Part model, mm, in its own coordinate system. A direction names the side the tool comes from. Round coordinates to 2 decimals unless told otherwise and drop trailing zeros. Loops run counter-clockwise (first coordinate to the right, second up) from the corner with the lowest first, then second, coordinate; pieces in that order, holes last. Notation, with made-up numbers: M 64.25,-15 L 120.25,-15 A24 ccw 120.25,13 Z; hole C -8,25.5 d4. An arc over 180 degrees is marked long. Put each result on its own line as item: value. Start each with the question number.
1) Slice it at B-B on x = 64.5. Give the cut face in (y, z).
2) Pull direction X, two halves, no side cores. Call faces 1 (the cylindrical face through (-11.797, -7.259, 11.668)), 2 (the cylindrical face through (-2.855, -4.31, 11.454)), 3 (the cylindrical face through (-3.01, -4.31, -18.15)), 4 (the cylindrical face through (-2.85, -4.31, 6.99)): +X half, -X half, draft (parallel to the pull), parting line (faces both ways), or undercut.
3) Drop flat-ended pins along their axis: pin 1 Ø1 at (x, y) = (60.5, -4) entering from -Z; pin 2 Ø2.5 at (y, z) = (-5.5, -3.5) entering from -X; pin 3 Ø5 at (x, y) = (95.5, -4) entering from +Z. Give the stop position or say it passes through.
4) Slice it at A-A on z = -5. Give the cut face in (x, y).
5) Which spindle directions (+Z, -Z, +X, -X, +Y, -Y) get a long thin tool onto all of the face, cutting with end or side? Do faces 5 (the flat face through (0, -4, -5)), 6 (the flat face through (-11.3, -4.3, 10)), 7 (the cylindrical face through (-11.22, -4.73, -20.26)), 8 (the flat face through (65, -4, 0)). Say none if no direction does.
6) Probe line 1 along X through (y, z) = (-1, -9); line 2 along Z through (x, y) = (89, -5.5); line 3 along X through (y, z) = (-6.75, -14). List the from-to ranges inside material, lowest first.
```python
from build123d import *

# Parameters (mm, degrees)
SKETCH1_W           = 11
SKETCH1_H           = 8.5
BOSS_EXTRUDE1_DEPTH = 120
BOSS_EXTRUDE3_START = -8.5
BOSS_EXTRUDE3_DEPTH = 8.5
FILLET5_R           = 10
FILLET6_R           = 5
SKETCH18_R          = 1.25
BOSS_EXTRUDE4_DEPTH = 1.5
SKETCH19_R          = 1.25
BOSS_EXTRUDE5_DEPTH = 1.5
REVOLVE9_ANGLE      = 180
REVOLVE10_ANGLE     = 180


with BuildPart() as part:
    # Sketch1 → Boss-Extrude1 (new body)
    with BuildSketch(Plane(origin=(0, 0, 0), x_dir=(0, 0, -1), z_dir=(1, 0, 0))):
        with Locations((5.5, -4.25)):
            Rectangle(SKETCH1_W, SKETCH1_H)
    extrude(amount=BOSS_EXTRUDE1_DEPTH)

    # Sketch17 → Boss-Extrude3 (add)
    with BuildSketch(Plane(origin=(0, 0, 0), x_dir=(1, 0, 0), z_dir=(0, 1, 0)).offset(BOSS_EXTRUDE3_START)):
        with BuildLine():
            Line((-10, -10), (-13.5, -10))
            Line((-13.5, -10), (-13.5, -13.5))
            Line((-13.5, -13.5), (-10, -13.5))
            ThreePointArc((-10, -13.5), (-0.454058454, -9.545941546), (3.5, 0))
            Line((3.5, 0), (3.5, 11))
            ThreePointArc((3.5, 11), (-0.454058454, 20.545941546), (-10, 24.5))
            Line((-10, 24.5), (-13.5, 24.5))
            Line((-13.5, 24.5), (-13.5, 21))
            Line((-13.5, 21), (-10, 21))
            ThreePointArc((-10, 21), (-2.928932188, 18.071067812), (0, 11))
            Line((0, 11), (0, 0))
            ThreePointArc((0, 0), (-2.928932188, -7.071067812), (-10, -10))
        make_face()
    extrude(amount=BOSS_EXTRUDE3_DEPTH)

    # Fillet5
    fillet5_edges = [part.edges().sort_by_distance(p)[0] for p in [
        (3.5, -4.25, 0),
        (3.5, -4.25, -11),
    ]]
    fillet(fillet5_edges, radius=FILLET5_R)

    # Fillet6
    # the kernel refuses this fillet: 5 mm, written as the material it takes off along each edge
    with BuildSketch(Plane(origin=(-13.5, -8.5, -2.5), x_dir=(0, 1, 0), z_dir=(0, 0, 1)), Plane(origin=(-13.5, 0, -2.5), x_dir=(1, 0, 0), z_dir=(0, 0, 1)), Plane(origin=(-13.5, -8.5, -37), x_dir=(0, 1, 0), z_dir=(0, 0, 1)), Plane(origin=(-13.5, 0, -37), x_dir=(1, 0, 0), z_dir=(0, 0, 1))) as fillet6_piece_1:
        with BuildLine():
            CenterArc((FILLET6_R, -FILLET6_R), FILLET6_R, 90, 90)
            Line((0, -FILLET6_R), (0, 0))
            Line((0, 0), (FILLET6_R, 0))
        make_face()
    extrude(amount=28.5, mode=Mode.SUBTRACT)

    # Sketch18 → Boss-Extrude4 (add)
    with BuildSketch(Plane.XY.offset(-21)):
        with Locations(Location((-10, -5, 0), (0, 0, 270))):
            Circle(SKETCH18_R)
    extrude(amount=BOSS_EXTRUDE4_DEPTH)

    # Sketch19 → Boss-Extrude5 (add)
    with BuildSketch(Plane(origin=(0, 0, 10), x_dir=(-1, 0, 0), z_dir=(0, 0, -1))):
        with Locations(Location((10, -3.5, 0), (0, 0, 269.999999996))):
            Circle(SKETCH19_R)
    extrude(amount=BOSS_EXTRUDE5_DEPTH)

    # Sketch24 → Revolve9 (revolve)
    with BuildSketch(Plane(origin=(0, 0, 8.5), x_dir=(-1, 0, 0), z_dir=(0, 0, -1))):
        with BuildLine():
            Line((10, -2.25), (10, -4.75))
            ThreePointArc((10, -4.75), (11.25, -3.5), (10, -2.25))
        make_face()
    revolve(axis=Axis((-10, -2.25, 8.5), (0, -1, 0)), revolution_arc=REVOLVE9_ANGLE)

    # Sketch25 → Revolve10 (revolve)
    with BuildSketch(Plane.XY.offset(-19.5)):
        with BuildLine():
            Line((-10, -3.75), (-10, -6.25))
            ThreePointArc((-10, -6.25), (-11.25, -5), (-10, -3.75))
        make_face()
    revolve(axis=Axis((-10, -3.75, -19.5), (0, 1, 0)), revolution_arc=REVOLVE10_ANGLE)


solid = part.part
```
Recorded:
1. outline: M -8.5,-11 L 0,-11 L 0,0 L -8.5,0 Z
2. face 1: -X half
2. face 2: +X half
2. face 3: undercut
2. face 4: undercut
3. pin 1: stops at z = -11
3. pin 2: stops at x = 0
3. pin 3: stops at z = 0
4. outline: M 0,-8.5 L 120,-8.5 L 120,0 L 0,0 Z
5. face 5: -X, +Y, -Y
5. face 6: -X
5. face 7: none
5. face 8: +Z, +X, +Y, -Y
6. line 1: x = 0 to 120
6. line 2: z = -11 to 0
6. line 3: x = -0.46 to 4.12
